```python
from build123d import *

# Parameters (mm, degrees)
SKETCH_1_R          = 40
SKETCH_1_R_2        = 33
EXTRUDE_1_DEPTH     = 4
EXTRUDE_START       = 8
SKETCH_2_R          = 40
SKETCH_2_R_2        = 36
EXTRUDE_2_DEPTH     = 8
EXTRUDE_3_DEPTH     = 3
SKETCH_6_R          = 2
CUT_EXTRUDE_1_DEPTH = 3
SKETCH_7_R          = 1.2
CUT_EXTRUDE_2_DEPTH = 5


with BuildPart() as part:
    # 草图1 → 凸台-拉伸1 (new body)
    with BuildSketch(Plane.XY):
        with Locations((-86.606649797, -63.783530386)):
            Circle(SKETCH_1_R)
        with Locations((-86.606649797, -63.783530386)):
            Circle(SKETCH_1_R_2, mode=Mode.SUBTRACT)
    extrude(amount=EXTRUDE_1_DEPTH)

    # 草图2 → 凸台-拉伸2 (add)
    with BuildSketch(Plane(origin=(0, 0, 0), x_dir=(-1, 0, 0), z_dir=(0, 0, -1)).offset(EXTRUDE_START)):
        with Locations((86.606649797, -63.783530386)):
            Circle(SKETCH_2_R)
        with Locations((86.606649797, -63.783530386)):
            Circle(SKETCH_2_R_2, mode=Mode.SUBTRACT)
    extrude(amount=-EXTRUDE_2_DEPTH)

    # 草图4 → 凸台-拉伸3 (add)
    with BuildSketch(Plane.XY.offset(4)):
        with BuildLine():
            Line((-102.470674133, 52.025849932), (-145.802574452, 37.009933401))
            Line((-145.802574452, 37.009933401), (-118.238289751, -42.533185695))
            ThreePointArc((-118.238289751, -42.533185695), (-99.084005703, -27.777233919), (-74.906389432, -27.517269163))
            Line((-74.906389432, -27.517269163), (-102.470674133, 52.025849932))
        make_face()
    extrude(amount=-EXTRUDE_3_DEPTH)

    # 草图6 → 切除-拉伸1 (cut)
    with BuildSketch(Plane(origin=(0, 0, 1), x_dir=(-1, 0, 0), z_dir=(0, 0, -1))):
        with Locations((120.302459735, 31.916433112)):
            Circle(SKETCH_6_R)
        with Locations((126.956233046, 18.205691171)):
            Circle(SKETCH_6_R)
        with Locations((106.591717794, 25.262659801)):
            Circle(SKETCH_6_R)
    extrude(amount=-CUT_EXTRUDE_1_DEPTH, mode=Mode.SUBTRACT)

    # 草图7 → 切除-拉伸2 (cut)
    with BuildSketch(Plane.XY.offset(4)):
        with Locations((-117.474470724, -5.248159683)):
            Circle(SKETCH_7_R)
        with Locations((-110.925868003, -24.145667519)):
            Circle(SKETCH_7_R)
        with Locations((-98.576962888, 1.300443037)):
            Circle(SKETCH_7_R)
        with Locations((-92.028360167, -17.597064799)):
            Circle(SKETCH_7_R)
    extrude(amount=-CUT_EXTRUDE_2_DEPTH, mode=Mode.SUBTRACT)


solid = part.part
```
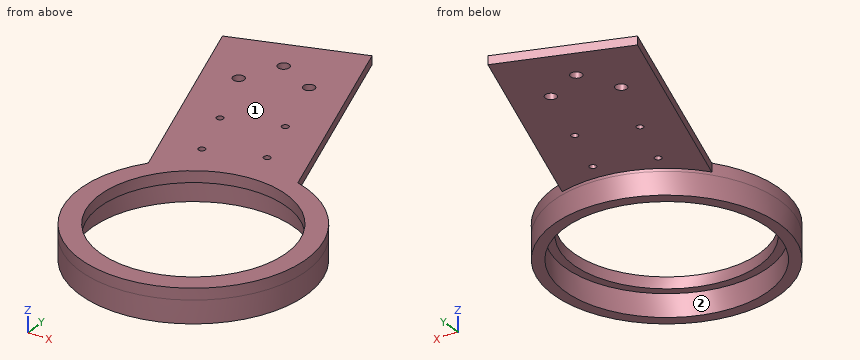
Design review of the part built by this model. Coordinates are the model's own, in mm. Face numbers are marked on the shaded views. Give positions to 0.01 mm unless a question says otherwise; leave off trailing zeros. Order: outer loops, then holes, each group sorted by start corner. A loop starts at its lowest first (then second) coordinate and runs counter-clockwise, first axis right, second up. Notation, with made-up numbers: M -31,-4 L -1,-4 A19 ccw -1,1 Z; hole C -38,51 d2. An arc over 180 degrees is marked long. One line per question, with ' | ' between items. Start each with the question number.
Q1. For pin 1 Ø3 at (x, y) = (-98.58, 1.3) entering from -Z; pin 2 Ø2.5 at (x, y) = (-120.3, 31.92) entering from +Z; pin 3 Ø1.5 at (x, z) = (-63, 2.5) entering from -Y; pin 4 Ø6.5 at (x, y) = (-126.96, 18.21) entering from +Z, all flat-tipped, find the tip position at first contact; note any pin that passes through.
Q2. We need section A-A (y = -42.5). Write out the cut boundary in (x, z).
Q3. We need section B-B (x = -68). Write out the cut boundary in (y, z).
Q4. We need section C-C (y = -9). Write out the cut boundary in (x, z).
Q5. We need section D-D (z = -5.25). Write out the cut boundary in (x, y), plus the area to 3 significant figures.
Q6. For L1, parallel to X at y = -61, z = 3.5; L2, parallel to Y at x = -112, z = -6; L3, parallel to X at y = -64, z = 1.25, list the stretches that pass through material, from the lowest coordinate up. Write a range as [from, to].
Q7. The part is to be moulded in two halves that separate along X. For the marked faces 1 and 2, say which applies: +X half, -X half, draft (parallel to the pull), parting line (faces both ways), or undercut.
Returned:
1) pin 1: z = 1 | pin 2: through | pin 3: y = -96.61 | pin 4: z = 4
2) outline: M -120.47,-8 L -115.64,-8 L -115.64,0 L -111.83,0 L -111.83,4 L -120.47,4 Z; M -61.39,0 L -57.57,0 L -57.57,-8 L -52.74,-8 L -52.74,4 L -61.39,4 Z
3) outline: M -99.19,-8 L -94.6,-8 L -94.6,0 L -91.04,0 L -91.04,4 L -99.19,4 Z; M -36.53,0 L -32.96,0 L -32.96,-8 L -28.37,-8 L -28.37,4 L -36.53,4 Z
4) outline: M -129.86,1 L -81.32,1 L -81.32,4 L -129.86,4 Z
5) outline: C -86.61,-63.78 d80; hole C -86.61,-63.78 d72 | area: 955 mm2
6) L1: [-126.51, -119.49], [-53.72, -46.7] | L2: [-94.69, -89.3], [-38.27, -32.88] | L3: [-126.61, -119.61], [-53.61, -46.61]
7) face 1: draft | face 2: undercut
